Part model, mm, in its own coordinate system. A direction names the side the tool comes from. Give positions to 0.01 mm unless a question says otherwise; leave off trailing zeros. Write each loop counter-clockwise with the first axis right and the second up, starting at its lowest first coordinate (ties: lowest second). Pieces come first, ordered by that corner, then holes. Notation, with made-up numbers: (39, 42.25) - (88, 42.25) arc R19 ccw to (88, 62.25) - close; hole circle Ø9 at (57.5, 79). An arc over 180 degrees is marked (long way). Answer as a JSON object with one key per item and string values. Group by question number.
```python
from build123d import *

# Parameters (mm, degrees)
ESQUISSE1_W                       = 42
ESQUISSE1_H                       = 42
BOSS_EXTRU_1_DEPTH                = 41
ESQUISSE2_R                       = 11
BOSS_EXTRU_2_DEPTH                = 2
BOSS_EXTRU_3_DEPTH                = 22
DIAM_TRE_DU_PER_AGE_3_0_3_1_D     = 3
DIAM_TRE_DU_PER_AGE_3_0_3_1_DEPTH = 4.8
DIAM_TRE_DU_PER_AGE_3_0_3_1_TIP   = 0.901290929
CHANFREIN1_SIZE                   = 4
ENL_V_START                       = 9
ENL_V_MAT_EXTRU_1_DEPTH           = 23.5
ESQUISSE5_R                       = 0.7
ESQUISSE5_R_2                     = 0.654723083
BOSS_EXTRU_4_DEPTH                = 10


with BuildPart() as part:
    # Esquisse1 → Boss.-Extru.1 (new body)
    with BuildSketch(Plane(origin=(0, 0, 0), x_dir=(1, 0, 0), z_dir=(0, 1, 0))):
        Rectangle(ESQUISSE1_W, ESQUISSE1_H)
    extrude(amount=BOSS_EXTRU_1_DEPTH)

    # Esquisse2 → Boss.-Extru.2 (add)
    with BuildSketch(Plane(origin=(0, 41, 0), x_dir=(1, 0, 0), z_dir=(0, 1, 0))):
        with Locations(Location((0, 0, 0), (0, 0, 270))):
            Circle(ESQUISSE2_R)
    extrude(amount=BOSS_EXTRU_2_DEPTH)

    # Esquisse3 → Boss.-Extru.3 (add)
    with BuildSketch(Plane(origin=(0, 43, 0), x_dir=(1, 0, 0), z_dir=(0, 1, 0))):
        with BuildLine():
            Line((-1.5, 2), (1.5, 2))
            ThreePointArc((1.5, 2), (0, -2.5), (-1.5, 2))
        make_face()
    extrude(amount=BOSS_EXTRU_3_DEPTH)

    # Diamètre du perçage Ø3.0 (3)1
    with Locations(Plane(origin=(0, 41, 0), x_dir=(1, 0, 0), z_dir=(0, 1, 0))):
        with Locations((-15.5, 15.5), (15.5, 15.5), (15.5, -15.5), (-15.5, -15.5)):
            Hole(DIAM_TRE_DU_PER_AGE_3_0_3_1_D / 2, depth=DIAM_TRE_DU_PER_AGE_3_0_3_1_DEPTH)
            with Locations((0, 0, -(DIAM_TRE_DU_PER_AGE_3_0_3_1_DEPTH + DIAM_TRE_DU_PER_AGE_3_0_3_1_TIP / 2))):  # 118° drill point
                Cone(0, DIAM_TRE_DU_PER_AGE_3_0_3_1_D / 2, DIAM_TRE_DU_PER_AGE_3_0_3_1_TIP, mode=Mode.SUBTRACT)

    # Chanfrein1
    chanfrein1_edges = [part.edges().sort_by_distance(p)[0] for p in [
        (-21, 20.5, -21),
        (21, 20.5, -21),
        (21, 20.5, 21),
        (-21, 20.5, 21),
    ]]
    chamfer(chanfrein1_edges, length=CHANFREIN1_SIZE)

    # Esquisse4 → Enlèv. mat.-Extru.1 (cut)
    with BuildSketch(Plane(origin=(0, 0, 0), x_dir=(1, 0, 0), z_dir=(0, 1, 0)).offset(ENL_V_START)):
        Polygon((-14, 21), (-21, 14), (-21, 21), align=None)
        Polygon((21, 21), (14, 21), (21, 14), align=None)
        Polygon((14, -21), (21, -14), (21, -21), align=None)
        Polygon((-21, -21), (-14, -21), (-21, -14), align=None)
    extrude(amount=ENL_V_MAT_EXTRU_1_DEPTH, mode=Mode.SUBTRACT)

    # Esquisse5 → Boss.-Extru.4 (add)
    with BuildSketch(Plane.ZY.offset(21)):
        with Locations(Location((-1, 7, 0), (0, 0, 180))):
            Circle(ESQUISSE5_R)
        with Locations(Location((-1, 5, 0), (0, 0, 180))):
            Circle(ESQUISSE5_R_2)
        with Locations(Location((1, 5, 0), (0, 0, 180))):
            Circle(ESQUISSE5_R_2)
        with Locations(Location((1, 7, 0), (0, 0, 180))):
            Circle(ESQUISSE5_R)
    extrude(amount=BOSS_EXTRU_4_DEPTH)


solid = part.part
```
1) Drop flat-ended pins along their axis: P1, Ø1.5, axis at y = 20.5, z = 15.5, coming from the +X side; P2, Ø1.5, axis at y = 24, z = -11.5, coming from the -X side; P3, Ø1, axis at x = -11.5, z = -6.5, coming from the +Y side; P4, Ø2.5, axis at x = 15.5, z = -15.5, coming from the -Y side. Give the stop position or say it passes through.
2) Drill centre lines: line 1 along X through (y, z) = (39.15, -15.5); line 2 along X through (y, z) = (39, -15). Where is each one in solid material? Low to high. Write a range as from..to.
3) Which spindle directions (+Z, -Z, +X, -X, +Y, -Y) get a long thin tool onto all of the face, cutting with end or side? Do faces 1 (the flat face through (-18, 32.5, -18)), 2 (the flat face through (17, 21, 18)), 3 (the cylindrical face through (-10.74, 41.99, -2.38)), 4 (the flat face through (17, 21, -18)). Say none if no direction does.
4) Saw through at A-A (x = 0). List the corners of the cut face in (y, z).
5) Saw through at C-C (z = 12.5). List the corners of the cut face in (x, y).
6) Two-plate mould, pull along X, no slides. Class faces 5 (the conical face through (-15.38, 35.455, 15.731)), 6 (the flat face through (21, 20, 0)), 7 (the cylindrical face through (-14, 38.57, -15.57)), 8 (the flat face through (0, 65, 0)): +X half, -X half, draft (parallel to the pull), parting line (faces both ways), or undercut.
7) Saw through at B-B (y = 30.5). List the corners of the cut face in (x, z), and give its area (3 significant figures).
8) Saw through at D-D (x = 5.5). List the corners of the cut face in (y, z).
Checks:
{
 "1": {"P1": "x = 20.25", "P2": "x = -21", "P3": "y = 41", "P4": "y = 0"},
 "2": {"line 1": "-21..-17, -14..14, 17..21", "line 2": "-21..-16.91, -14.09..14.09, 16.91..21"},
 "3": {"face 1": "-Z, -X", "face 2": "+Z, +X", "face 3": "+Y", "face 4": "-Z, +X"},
 "4": {"outline": "(0, -21) - (41, -21) - (41, -11) - (43, -11) - (43, -2) - (65, -2) - (65, 2.5) - (43, 2.5) - (43, 11) - (41, 11) - (41, 21) - (0, 21) - close"},
 "5": {"outline": "(-21, 0) - (21, 0) - (21, 41) - (-21, 41) - close"},
 "6": {"face 5": "undercut", "face 6": "+X half", "face 7": "undercut", "face 8": "draft"},
 "7": {"outline": "(-21, -14) - (-14, -21) - (14, -21) - (21, -14) - (21, 14) - (14, 21) - (-14, 21) - (-21, 14) - close", "area": "1,670 mm2"},
 "8": {"outline": "(0, -21) - (41, -21) - (41, -9.53) - (43, -9.53) - (43, 9.53) - (41, 9.53) - (41, 21) - (0, 21) - close"}
}
